```python
from build123d import *

# Parameters (mm, degrees)
BOSS_EXTRUDE1_DEPTH = 2


with BuildPart() as part:
    # Sketch1 → Boss-Extrude1 (new body)
    with BuildSketch(Plane.XY):
        with BuildLine():
            Line((-37.821244, 0.214456948), (-37.821244, 0))
            Line((-37.821244, 0), (-37.821244, -6))
            ThreePointArc((-37.821244, -6), (-37.235457562, -7.414213562), (-35.821244, -8))
            Line((-35.821244, -8), (-21.821244, -8))
            Line((-21.821244, -8), (-21.821244, 5.35))
            Line((-21.821244, 5.35), (-32.821244, 5.35))
            Line((-32.821244, 5.35), (-32.821244, 6.35))
            Line((-32.821244, 6.35), (-37.821244, 6.35))
            Line((-37.821244, 6.35), (-37.821244, 4))
            Line((-37.821244, 4), (-37.821244, 1))
            Line((-37.821244, 1), (-37.821244, 0.587709258))
            Line((-37.821244, 0.587709258), (-37.821244, 0.214456948))
        make_face()
    extrude(amount=BOSS_EXTRUDE1_DEPTH)


solid = part.part
```
Could you check a few things on this model? Use its own coordinates, in mm. A direction names the side the tool comes from. Give positions to 0.01 mm unless a question says otherwise; leave off trailing zeros. Order: outer loops, then holes, each group sorted by start corner. A loop starts at its lowest first (then second) coordinate and runs counter-clockwise, first axis right, second up.
Q1. I'm going to push a flat-ended pin straight in: P1, Ø0.5, axis at y = 6, z = 1, coming from the +X side. Where does the tip first touch, or does it pass through?
Q2. Suppose I cut it at A-A, the plane z = 0.6. Write out the boundary of the cut face in (x, y).
Q3. For faces 1 (the flat face through (-27, 5.35, 1)), 2 (the flat face through (-29, -8, 1)), which set-ups out of +Z, -Z, +X, -X, +Y, -Y let a thin tool reach every point of the face, with its end or its side?
Q4. Suppose I cut it at B-B, the plane x = -23. Write out the boundary of the cut face in (y, z), and give its area (3 significant figures).
Q5. If I drill on line 1 along X through (y, z) = (5.75, 1.25); line 2 along Y through (x, z) = (-25.25, 0.4); line 3 along Y through (x, z) = (-36.5, 1.75), over which ranges is the centre line in solid material (lowest first)?
Solution:
1. P1: stops at x = -32.82
2. outline: (-37.82, -6) arc R2 ccw to (-35.82, -8) - (-21.82, -8) - (-21.82, 5.35) - (-32.82, 5.35) - (-32.82, 6.35) - (-37.82, 6.35) - close
3. face 1: +Z, -Z, +X, +Y
3. face 2: +Z, -Z, +X, -X, -Y
4. outline: (-8, 0) - (5.35, 0) - (5.35, 2) - (-8, 2) - close
4. area: 26.7 mm2
5. line 1: x = -37.82 to -32.82
5. line 2: y = -8 to 5.35
5. line 3: y = -7.88 to 6.35
